Build history of the part. All positions in model axes, mm. A direction names the side the tool comes from. Give positions to 0.01 mm unless a question says otherwise; leave off trailing zeros. Loops run counter-clockwise (first coordinate to the right, second up) from the corner with the lowest first, then second, coordinate; pieces in that order, holes last.
1) Band-saw the part on A-A on z = -0.75. List the corners of the cut face in (x, y), then the cut area to 3 significant figures.
2) Two-plate mould, pull along X, no slides. Class faces 4 (the cylindrical face through (-5.01, 4.25, -3.13)), 5 (the flat face through (-1, 10.6, 16.1)), 6 (the flat face through (0, 0, 0)), 7 (the cylindrical face through (6.99, 4.25, -3.13)): +X half, -X half, draft (parallel to the pull), parting line (faces both ways), or undercut.
3) Wall check: line 1 (Y direction, x = 8.5, z = 3.5); line 2 (Y direction, x = 0, z = 12.5); line 3 (Z direction, x = 2.75, y = 1). Give the ranges that are in metal, low to high.
4) Band-saw the part on B-B on x = -0.5. List the corners of the cut face in (y, z).
5) Flat gauge pins, fed straight in: P1, Ø5, axis at x = 2, z = 4, coming from the +Y side; P2, Ø2, axis at x = 0, y = 19.5, coming from the -Z side; P3, Ø8, axis at y = 17.5, z = 11, coming from the +X side. Where does each tip first touch, or does it go through?
6) Band-saw the part on D-D on x = -3.75. List the corners of the cut face in (y, z), then the cut area to 3 significant figures.
7) 3-axis set-ups, long thin cutter, end or side, ignore diameter. For faces 1 (the cylindrical face through (-3.59, 2.99, 0.07)), 2 (the flat face through (1, 10.6, 16.1)), 3 (the cylindrical face through (0.079, 2.986, -3.646)): which of +Z, -Z, +X, -X, +Y, -Y reach the whole face in a straight line?
8) Band-saw the part on C-C on y = 13. List the corners of the cut face in (x, z), then the cut area to 3 significant figures.
```python
from build123d import *

# Parameters (mm, degrees)
SKETCH1_W           = 20
SKETCH1_H           = 16
BOSS_EXTRUDE1_DEPTH = 2
SKETCH2_R           = 1
BOSS_EXTRUDE2_DEPTH = 2
BOSS_EXTRUDE3_DEPTH = 1
SKETCH10_R          = 1
BOSS_EXTRUDE4_DEPTH = 2.5


with BuildPart() as part:
    # Sketch1 → Boss-Extrude1 (new body)
    with BuildSketch(Plane(origin=(0, 0, 0), x_dir=(1, 0, 0), z_dir=(0, 1, 0))):
        Rectangle(SKETCH1_W, SKETCH1_H)
    extrude(amount=BOSS_EXTRUDE1_DEPTH)

    # Sketch2 → Boss-Extrude2 (add)
    with BuildSketch(Plane(origin=(0, 2, 0), x_dir=(1, 0, 0), z_dir=(0, 1, 0))):
        with BuildLine():
            Line((-1, -2.469823306), (-1, -7.190883186))
            Line((-1, -7.190883186), (1, -7.190883186))
            Line((1, -7.190883186), (1, -2.469823306))
            ThreePointArc((1, -2.469823306), (3.552605477, -0.099588475), (6.583085105, 1.617968249))
            ThreePointArc((6.583085105, 1.617968249), (7.413613283, 3.501694616), (5.581395349, 4.440406243))
            ThreePointArc((5.581395349, 4.440406243), (0, 3.645822822), (-5.581395349, 4.440406243))
            ThreePointArc((-5.581395349, 4.440406243), (-7.413613283, 3.501694616), (-6.583085105, 1.617968249))
            ThreePointArc((-6.583085105, 1.617968249), (-3.552605477, -0.099588475), (-1, -2.469823306))
        make_face()
        with Locations(Location((-6, 3, 0), (0, 0, 270))):
            Circle(SKETCH2_R, mode=Mode.SUBTRACT)
        with Locations(Location((6, 3, 0), (0, 0, 270))):
            Circle(SKETCH2_R, mode=Mode.SUBTRACT)
    extrude(amount=BOSS_EXTRUDE2_DEPTH)

    # Sketch8 → Boss-Extrude3 (add, symmetric)
    with BuildSketch(Plane(origin=(0, 0, 0), x_dir=(0, 0, -1), z_dir=(1, 0, 0))):
        with BuildLine():
            Line((-7.190883186, 4), (-7.190883186, 2))
            ThreePointArc((-7.190883186, 2), (-18.190883186, 13), (-7.190883186, 24))
            ThreePointArc((-7.190883186, 24), (-6.40597694, 23), (-7.190883186, 22))
            ThreePointArc((-7.190883186, 22), (-16.190883186, 13), (-7.190883186, 4))
        make_face()
    extrude(amount=BOSS_EXTRUDE3_DEPTH, both=True)

    # Sketch10 → Boss-Extrude4 (add)
    with BuildSketch(Plane(origin=(0, 2, 0), x_dir=(1, 0, 0), z_dir=(0, 1, 0))):
        with Locations(Location((6, 3, 0), (0, 0, 270))):
            Circle(SKETCH10_R)
        with Locations(Location((-6, 3, 0), (0, 0, 270))):
            Circle(SKETCH10_R)
    extrude(amount=BOSS_EXTRUDE4_DEPTH)


solid = part.part
```
Findings below:
1. outline: (-10, 0) - (10, 0) - (10, 2) - (4.85, 2) - (4.85, 4) - (-4.85, 4) - (-4.85, 2) - (-10, 2) - close
1. area: 59.4 mm2
2. face 4: undercut
2. face 5: -X half
2. face 6: draft
2. face 7: undercut
3. line 1: y = 0 to 2
3. line 2: y = 3.37 to 5.73, 20.27 to 22.63
3. line 3: z = -8 to 8
4. outline: (0, -8) - (2, -8) - (2, -3.65) - (4, -3.65) - (4, 7.19) arc R9 cw to (22, 7.19) arc R1.03 ccw to (24, 7.19) arc R11 ccw to (2, 7.19) - (2, 8) - (0, 8) - close
5. P1: stops at y = 4
5. P2: stops at z = 12.17
5. P3: stops at x = 1
6. outline: (0, -8) - (2, -8) - (2, -4) - (4, -4) - (4, -0.04) - (2, -0.04) - (2, 8) - (0, 8) - close
6. area: 39.9 mm2
7. face 1: +Z, -X, +Y
7. face 2: +Z, +X, +Y
7. face 3: -Z, +Y
8. outline: (-1, 16.19) - (1, 16.19) - (1, 18.19) - (-1, 18.19) - close
8. area: 4.00 mm2
